Source: CAD feature listing. Evaluate the final solid. Frame: model axes, mm. Give positions to 0.01 mm unless a question says otherwise; leave off trailing zeros. Order: outer loops, then holes, each group sorted by start corner. A loop starts at its lowest first (then second) coordinate and runs counter-clockwise, first axis right, second up. Notation, with made-up numbers: M 49,-31.5 L 100,-31.5 A23 cw 100,-11.5 Z; hole C 30,-7.75 d5. An arc over 180 degrees is marked long. Answer in a Markdown table with one row per item. Add a question column.
(1) Mould query, pull axis Y, two halves, no side actions, for faces 1 (the face through (1.578, 3.982, -1.254)), 2 (the face through (1.62, -0.1, -36.14)), 3 (the face through (1.622, -85.215, 0.136)). Classes: pulls with the +Y half, pulls with the -Y half, needs draft (parallel to the pull), parting line crosses it, or undercut.
(2) Section query D-D, the plane y = -32.5. Return loops of the section in (x, z), plus the area to 3 significant figures.
(3) Section query C-C, the plane z = 25. Return loops of the section in (x, y).
(4) Section query A-A, the plane y = 0. Return loops of the section in (x, z) (3 decimals).
(5) Section query B-B, the plane x = 1.4. Return loops of the section in (y, z) (3 decimals), plus the area to 3 significant figures.
(6) Material intervals for line 1 along Y through (x, z) = (2.95, 1); line 2 along Z through (x, y) = (2.4, -12.5); line 3 along Z through (x, y) = (1.95, 0) (3 decimals), sorted ascending.
Autodesk Inventor part; units mm, degrees
ref_plane "YZ Plane" through (0, 0, 0) normal (1, 0, 0) x (0, 1, 0)
ref_plane "XZ Plane" through (0, 0, 0) normal (0, 1, 0) x (-1, 0, 0)
ref_plane "XY Plane" through (0, 0, 0) normal (0, 0, 1) x (1, 0, 0)
sketch "Sketch1" plane through (0, 0, 0) normal (1, 0, 0) x (0, 1, 0)
  line L0 (-122.5, 0) -> (122.5, 0) construction
  line L1 (0, -52.5) -> (0, 52.5) construction
  line L2 (-100, 0) -> (0, 37.5)
  line L3 (0, 37.5) -> (100, 0)
  line L4 (100, 0) -> (0, -37.5)
  line L5 (-100, 0) -> (0, -37.5)
  circle A0 centre (0, 0) radius 4.175
  circle A1 centre (25, 0) radius 0.75
  line L6 (25, 0) -> (-12.5, -21.6506) construction
  line L7 (-12.5, -21.6506) -> (-12.5, 21.6506) construction
  line L8 (-12.5, 21.6506) -> (25, 0) construction
  circle A2 centre (-12.5, 21.6506) radius 0.75
  circle A3 centre (-12.5, -21.6506) radius 0.75
  circle A4 centre (0, 0) radius 25 construction
  dimension "d7" = 50
  dimension "d3" = 8.35
  dimension "d4" = 1.5
  dimension "d11" = 75
  dimension "d24" = 200
extrude "Extrusion1" add sketch "Sketch1" along normal blind 3.2
fillet "Fillet1" radius 20 2 edges at (1.6, 0, 37.5) (1.6, 0, -37.5)
sketch "Sketch4" plane through (3.2, 0, 0) normal (1, 0, 0) x (0, 0, -1)
  circle A0 centre (0, 0) radius 4.175
  circle A1 centre (0, -7.9) radius 1.425
  dimension "d20" = 7.9
  dimension "d21" = 2.85
extrude "Extrusion4" cut sketch "Sketch4" against normal through all contours A1
fillet "Fillet4" radius 8 2 edges at (1.6, 100, 0) (1.6, -100, 0)
sketch "Sketch5" plane through (0, 0, 0) normal (-1, 0, 0) x (0, 0, 1)
  circle A0 centre (-21.6506, -12.5) radius 0.75
  circle A1 centre (-2.0715, -16.5813) radius 1.425
  line L0 (-2.0715, -16.5813) -> (-21.6506, -12.5) construction
  circle A2 centre (0, -7.9) radius 1.425
  circle A3 centre (0, 0) radius 4.175
  circle A4 centre (-2.0715, -16.5813) radius 7.5 construction
  line L1 (-2.0715, -16.5813) -> (7.7181, -18.6219) construction
  circle A5 centre (7.7181, -18.6219) radius 1.425
  circle A6 centre (15.3955, 6.4967) radius 1.425
  circle A7 centre (12.268, 15.995) radius 1.425
  circle A8 centre (-13.3241, 10.0846) radius 1.425
  circle A9 centre (-19.9861, 2.6269) radius 1.425
  point P0 (22.1831, -13.0282)
  point P1 (-22.1831, -13.0282)
  dimension "d31" = 2.85
  dimension "d32" = 20
  dimension "d33" = 15
  dimension "d38" = 10
  dimension "d41" = 360
sketch "Sketch3" plane through (3.2, 0, 0) normal (1, 0, 0) x (0, 0, -1)
  line L0 (-7.7286, 24.361) -> (0, 66.8014)
  line L1 (0, 66.8014) -> (7.7286, 24.361)
  line L2 (8.0286, -24.361) -> (0, -68.4486)
  line L3 (0, -68.4486) -> (-8.0286, -24.361)
  line L4 (-7.7286, 24.361) -> (7.7286, 24.361)
  line L5 (-8.0286, -24.361) -> (8.0286, -24.361)
  line L6 (52.5, 0) -> (-52.5, 0)
sketch "Sketch2" plane through (3.2, 0, 0) normal (1, 0, 0) x (0, 0, -1)
  circle A0 centre (0, 0) radius 4.175
  circle A1 centre (0, 0) radius 3.048
  dimension "d13" = 6.096
equation "\"d24\" = Height"
equation "\"Height\" = 200"
properties part number "RibSimple"
Values follow:
| question | item | result |
|---|---|---|
| 1 | face 1 | undercut |
| 1 | face 2 | parting line crosses it |
| 1 | face 3 | pulls with the -Y half |
| 2 | outline | M 0,-25.31 L 3.2,-25.31 L 3.2,25.31 L 0,25.31 Z |
| 2 | area | 162 mm² |
| 3 | outline | M 0,-33.33 L 3.2,-33.33 L 3.2,33.33 L 0,33.33 Z |
| 4 | outline | M 0,-36.14 L 3.2,-36.14 L 3.2,-4.175 L 0,-4.175 Z; M 0,4.175 L 3.2,4.175 L 3.2,36.14 L 0,36.14 Z |
| 5 | outline | M -80.025,-7.491 L -7.022,-34.867 A20 ccw 7.022,-34.867 L 80.025,-7.491 A8 ccw 80.025,7.491 L 7.022,34.867 A20 ccw -7.022,34.867 L -80.025,7.491 A8 ccw Z; hole C -12.5,-21.651 d1.5; hole C -12.5,21.651 d1.5; hole C -7.9,0 d2.85; hole C 0,0 d8.35; hole C 25,0 d1.5 |
| 5 | area | 7,230 mm² |
| 6 | line 1 | y = -85.15 to -8.92, -6.88 to -4.05, 4.05 to 85.15 |
| 6 | line 2 | z = -32.81 to -22.4, -20.9 to 20.9, 22.4 to 32.81 |
| 6 | line 3 | z = -36.14 to -4.175, 4.175 to 36.14 |
